from build123d import *

# Parameters (mm, degrees)
F1_DEPTH = 12.7
F0_R     = 37.1561750652
F2_DEPTH = 50.8
F3_W     = 62.4604108743
F3_H     = 23.1594787911
F4_DEPTH = 38.1
F6_DEPTH = 25.4


with BuildPart() as f1:
    # F0 (on Top) → F1 (new body)
    with BuildSketch(Plane.XY):
        with BuildLine():
            Line((23.0791009963, 65.5601993203), (-73.9074721932, 65.5601993203))
            Line((-73.9074721932, 65.5601993203), (-73.9074721932, -34.29678455))
            Line((-73.9074721932, -34.29678455), (23.0791009963, -34.29678455))
            ThreePointArc((23.0791009963, -34.29678455), (-8.0472334197, 15.6317073852), (23.0791009963, 65.5601993203))
        make_face()
    extrude(amount=F1_DEPTH)

    # F0 (on Top) → F2 (join)
    with BuildSketch(Plane.XY):
        with BuildLine():
            ThreePointArc((103.1673720276, 15.6317073852), (76.978188725, 62.8201208563), (23.0791009963, 65.5601993203))
            ThreePointArc((23.0791009963, 65.5601993203), (-8.0472334197, 15.6317073852), (23.0791009963, -34.29678455))
            ThreePointArc((23.0791009963, -34.29678455), (76.978188725, -31.556706086), (103.1673720276, 15.6317073852))
        make_face()
        with Locations((47.5600693039, 15.6317073852)):
            Circle(F0_R, mode=Mode.SUBTRACT)
    extrude(amount=F2_DEPTH)

    # F3 (on Top) → F4 (join)
    with BuildSketch(Plane.XY):
        with Locations((-23.632629076, 15.6614030711)):
            Rectangle(F3_W, F3_H)
    extrude(amount=F4_DEPTH)

    # F5 (on face) → F6 (cut)
    with BuildSketch(Plane.XZ.offset(-4.0816636756)):
        Polygon((-54.8628345132, 38.1), (-54.8628345132, 12.7), (-6.8344948225, 38.1), align=None)
    extrude(amount=-F6_DEPTH, mode=Mode.SUBTRACT)


solid = f1.part
Here's how the part is built. I have some questions about the finished solid (model axes, mm). A direction names the side the tool comes from. Coordinates: 2 decimals unless noted, no trailing zeros. Loops run counter-clockwise (first coordinate to the right, second up) from the corner with the lowest first, then second, coordinate; pieces in that order, holes last. Notation, with made-up numbers: (-10, 45) -> (0, 45) arc R18 ccw to (0, 75) -> close; hole circle Ø11 at (66, 81). An arc over 180 degrees is marked (long way). Use one line per item in the form item = value. Start each with the question number.
(1) Will these pins go through, and if not, where does the flat tip stop? pin 1 (7.5 mm diameter, centred on x = -23, z = 24.5, fed in from +Y); pin 2 (4 mm diameter, centred on x = -7.5, z = 9.5, fed in from +Y); pin 3 (2 mm diameter, centred on y = 10.5, z = 44.5, fed in from -X); pin 4 (1.3 mm diameter, centred on x = -7.5, y = 18.5, fed in from -Z).
(2) If we section it at A-A (x = 30.5): Please give me the cut outline in (y, z), then the cut area to 3 significant figures.
(3) If we section it at C-C (y = 24): Please give me the cut outline in (x, z), then the cut area to 3 significant figures.
(4) We'd pull the mould along Y, two halves only. Please class faces 4 (the face through (-21, 4.082, 20)), 5 (the face through (59, -21, 50.8)), 6 (the face through (20.17, 40.74, 25.04)): pulls with the +Y half, pulls with the -Y half, needs draft (parallel to the pull), parting line crosses it, or undercut.
(5) Please list where these lines run through material, in increasing order: line 1 along X through (y, z) = (17, 39.5); line 2 along Y through (x, z) = (43.5, 42); line 3 along Z through (x, y) = (-59.5, -29).
(6) On a 3-axis mill with a long thin cutter (end or side, diameter ignored), from which of +Z, -Z, +X, -X, +Y, -Y can I reach the whole of each face in a straight line? I mean faces 1 (the face through (-25, 65.56, 6)), 2 (the face through (-36.9, 27.4, 12.7)), 3 (the face through (-26, 27.241, 22)). Say none if no direction works.
(7) If we section it at B-B (z = 5.5): Please give me the cut outline in (x, y), then the cut area to 3 significant figures.
(8) If we section it at D-D (x = 0): Please give me the cut outline in (y, z), then the cut area to 3 significant figures.
Verdict:
q1.pin_1 = 27.24
q1.pin_2 = 65.56
q1.pin_3 = -7.89
q1.pin_4 = 0
q2.outline = (-37.29, 0) -> (-17.38, 0) -> (-17.38, 50.8) -> (-37.29, 50.8) -> close; (48.64, 0) -> (68.56, 0) -> (68.56, 50.8) -> (48.64, 50.8) -> close
q2.area = 2,020 mm²
q3.outline = (-73.91, 0) -> (11.36, 0) -> (11.36, 50.8) -> (-7.41, 50.8) -> (-7.41, 38.1) -> (-6.83, 38.1) -> (-54.86, 12.7) -> (-73.91, 12.7) -> close; (83.76, 0) -> (102.53, 0) -> (102.53, 50.8) -> (83.76, 50.8) -> close
q3.area = 3,350 mm²
q4.face_4 = pulls with the -Y half
q4.face_5 = needs draft
q4.face_6 = undercut
q5.line_1 = -8.03 to 10.43, 84.69 to 103.15
q5.line_2 = -39.83 to -21.3, 52.57 to 71.09
q5.line_3 = 0 to 12.7
q6.face_1 = +Z, -Z, -X, +Y
q6.face_2 = +Z, -X
q6.face_3 = +Z, -X, +Y
q7.outline = (-73.91, -34.3) -> (23.08, -34.3) arc R55.61 ccw (long way) to (23.08, 65.56) -> (-73.91, 65.56) -> close; hole circle Ø74.31 at (47.56, 15.63)
q7.area = 12,800 mm²
q8.outline = (-34.3, 0) -> (65.56, 0) -> (65.56, 12.7) -> (44.45, 12.7) -> (44.45, 50.8) -> (-13.18, 50.8) -> (-13.18, 12.7) -> (-34.3, 12.7) -> close
q8.area = 3,460 mm²
